Geometry check sheet. Reference: the model listing, model coordinates, mm. A direction names the side the tool comes from. Round coordinates to 2 decimals unless told otherwise and drop trailing zeros. Order: outer loops, then holes, each group sorted by start corner. A loop starts at its lowest first (then second) coordinate and runs counter-clockwise, first axis right, second up. Notation, with made-up numbers: (-13.5, 15) - (24.5, 15) arc R22 cw to (24.5, 29) - close; hole circle Ø6 at (79.5, 40.5). An arc over 180 degrees is marked (long way). Use a Markdown table: item, result. Add a question column.
(1) Thickness scan on line 1 along X through (y, z) = (-2, 0); line 2 along X through (y, z) = (-0.75, 29). Record the ranges inside material, lowest first. Write a range as [from, to].
(2) Mould release check, pull along X, two halves, no side actions. Record for faces 1 (the face through (41.275, 5, -53)), 2 (the face through (-68.64, 0.09, -3.02)), 3 (the face through (-55, 6.35, 37)): released by +X, released by -X, zero draft, split by the parting line, or undercut.
(3) Section check B-B on x = 0. Record the boundary of the cut face in (y, z) (3 decimals), then the cut area to 3 significant figures.
(4) Access from +Z, -Z, +X, -X, +Y, -Y to the whole of each face (thin tool, end or side, straight path). Record for faces 4 (the face through (55, 6.35, 37)), 5 (the face through (55, 6.35, -37)), 6 (the face through (-41.275, 5, -53)), 7 (the face through (66, 12.446, 0)).
(5) Gauge pin test, flat ends, axial feed: P1, Ø2.5, axis at x = -63.5, y = 10.5, coming from the -Z side; P2, Ø1.6, axis at y = 4.5, z = 52, coming from the -X side; P3, Ø20, axis at x = 58.5, z = -44, coming from the +Y side; P4, Ø1.5, axis at y = 7.5, z = -21.5, coming from the +X side. Record the tip position at first contact, or that the pin passes through.
(6) Section check A-A on z = 0. Record the boundary of the cut face in (x, y), then the cut area to 3 significant figures.
```python
from build123d import *

# Parameters (mm, degrees)
SKETCH1_R           = 68.707
SKETCH1_R_2         = 65.532
BOSS_EXTRUDE1_DEPTH = 6.35
CUT_EXTRUDE1_DEPTH  = 3.175
BOSS_EXTRUDE2_DEPTH = 6.096


with BuildPart() as part:
    # Sketch1 → Boss-Extrude1 (new body, symmetric)
    with BuildSketch(Plane(origin=(0, 0, 0), x_dir=(1, 0, 0), z_dir=(0, 1, 0))):
        Circle(SKETCH1_R)
        Circle(SKETCH1_R_2, mode=Mode.SUBTRACT)
    extrude(amount=BOSS_EXTRUDE1_DEPTH, both=True)

    # Sketch2 → Cut-Extrude1 (cut)
    with BuildSketch(Plane(origin=(0, 6.35, 0), x_dir=(1, 0, 0), z_dir=(0, 1, 0))):
        with BuildLine():
            Line((-41.275, -50.900073), (-41.275, -54.927463))
            ThreePointArc((-41.275, -54.927463), (0, -68.707), (41.275, -54.927463))
            Line((41.275, -54.927463), (41.275, -50.900073))
            ThreePointArc((41.275, -50.900073), (0, -65.532), (-41.275, -50.900073))
        make_face()
    cut_extrude1 = extrude(amount=-CUT_EXTRUDE1_DEPTH, mode=Mode.SUBTRACT)

    # Mirror1: Cut-Extrude1 across plane
    add(cut_extrude1.mirror(Plane.XY), mode=Mode.SUBTRACT)

    # Sketch4 → Boss-Extrude2 (add)
    with BuildSketch(Plane(origin=(0, 6.35, 0), x_dir=(1, 0, 0), z_dir=(0, 1, 0))):
        with BuildLine():
            Line((-62.740442, 18.923), (-66.049769, 18.923))
            ThreePointArc((-66.049769, 18.923), (-68.707, 0), (-66.049769, -18.923))
            Line((-66.049769, -18.923), (-62.740442, -18.923))
            ThreePointArc((-62.740442, -18.923), (-65.532, 0), (-62.740442, 18.923))
        make_face()
    boss_extrude2 = extrude(amount=BOSS_EXTRUDE2_DEPTH)

    # Mirror3: Boss-Extrude2 across plane
    add(boss_extrude2.mirror(Plane(origin=(0, 0, 0), x_dir=(0, 0, 1), z_dir=(1, 0, 0))))


solid = part.part
```
Check sheet entries:
| question | item | result |
|---|---|---|
| 1 | line 1 | x = [-68.71, -65.53], [65.53, 68.71] |
| 1 | line 2 | x = [-62.29, -58.77], [58.77, 62.29] |
| 2 | face 1 | undercut |
| 2 | face 2 | split by the parting line |
| 2 | face 3 | zero draft |
| 3 | outline | (-6.35, -68.707) - (3.175, -68.707) - (3.175, -65.532) - (-6.35, -65.532) - close; (-6.35, 65.532) - (3.175, 65.532) - (3.175, 68.707) - (-6.35, 68.707) - close |
| 3 | area | 60.5 mm2 |
| 4 | face 4 | +Z, +X, -X, +Y |
| 4 | face 5 | -Z, +X, -X, +Y |
| 4 | face 6 | +Z, -Z, +Y |
| 4 | face 7 | +Z, -Z, +X, -X, +Y |
| 5 | P1 | stops at z = -18.92 |
| 5 | P2 | stops at x = -45.82 |
| 5 | P3 | stops at y = 6.35 |
| 5 | P4 | passes through |
| 6 | outline | (-68.71, -6.35) - (-65.53, -6.35) - (-65.53, 12.45) - (-68.71, 12.45) - close; (65.53, -6.35) - (68.71, -6.35) - (68.71, 12.45) - (65.53, 12.45) - close |
| 6 | area | 119 mm2 |
